from build123d import *

# Parameters (mm, degrees)
EXTRUDE_1_DEPTH          = 42.5
SKETCH_3_R               = 15
EXTRUDE_2_DEPTH          = 22
CUT_EXTRUDE_1_DEPTH      = 101.5
CUT_EXTRUDE_1_DEPTH_BACK = 101.5
FILLET_1_R               = 3
SKETCH_5_R               = 7.5
CUT_EXTRUDE_2_DEPTH      = 202


with BuildPart() as part:
    # 草图1 → 凸台-拉伸1 (new body, symmetric)
    with BuildSketch(Plane(origin=(0, 0, 0), x_dir=(0, 0, -1), z_dir=(1, 0, 0))):
        Polygon((-100.5, 100), (-42.5, 0), (42.5, 0), (100.5, 100), (100.5, 120), (95.5, 120), (95.5, 115), (95.5, 101.345066218), (39.619861593, 5), (-39.619861593, 5), (-95.5, 101.345066218), (-95.5, 115), (-95.5, 120), (-100.5, 120), align=None)
    extrude(amount=EXTRUDE_1_DEPTH, both=True)

    # 草图3 → 凸台-拉伸2 (add)
    with BuildSketch(Plane.XZ):
        Circle(SKETCH_3_R)
    extrude(amount=EXTRUDE_2_DEPTH)

    # 草图4 → 切除-拉伸1 (cut, two sides)
    with BuildSketch(Plane.XY) as cut_extrude_1_sk:
        Polygon((0, 78.450873214), (-15, 18.450873214), (15, 18.450873214), align=None)
    extrude(amount=CUT_EXTRUDE_1_DEPTH, mode=Mode.SUBTRACT)
    extrude(cut_extrude_1_sk.sketch, amount=-CUT_EXTRUDE_1_DEPTH_BACK, mode=Mode.SUBTRACT)

    # 圆角1
    fillet_1_edges = [part.edges().sort_by_distance(p)[0] for p in [
        (0, 78.450873214, -85.111437261),
        (0, 78.450873214, 85.111437261),
        (15, 18.450873214, -50.311437261),
        (15, 18.450873214, 50.311437261),
        (-15, 18.450873214, -50.311437261),
        (-15, 18.450873214, 50.311437261),
    ]]
    fillet(fillet_1_edges, radius=FILLET_1_R)

    # 草图5 → 切除-拉伸2 (cut, through all)
    with BuildSketch(Plane.XY.offset(100.5)):
        with Locations((0, 94)):
            Circle(SKETCH_5_R)
    extrude(amount=-CUT_EXTRUDE_2_DEPTH, mode=Mode.SUBTRACT)


solid = part.part
Input: part model. Units: mm. Frame: model coordinates. A direction names the side the tool comes from. Give positions to 0.01 mm unless a question says otherwise; leave off trailing zeros. Loops run counter-clockwise (first coordinate to the right, second up) from the corner with the lowest first, then second, coordinate; pieces in that order, holes last. Notation, with made-up numbers: (64, 69) -> (107, 69) arc R10 ccw to (107, 74) -> close; hole circle Ø7 at (17.5, 13.25). An arc over 180 degrees is marked (long way). Answer as a JSON object with one key per item and string values. Group by question number.
Item 1: Cut plane D-D, the plane x = 24. Return the cut outline in (y, z), and give its area (3 significant figures).
Item 2: Pin query (flat end, axial travel): P1, Ø1, axis at x = 24.5, z = 22, coming from the -Y side; P2, Ø1.5, axis at x = 25.5, y = 25, coming from the -Z side (3 decimals); P3, Ø3, axis at x = 13.5, y = 74, coming from the -Z side; P4, Ø12, axis at x = 0, y = 94, coming from the -Z side. Return the tip coordinate at first contact, or that it passes through.
Item 3: Reachability of faces 4 (the flat face through (1, 111, 95.5)), 5 (the cylindrical face through (6.93, 91.13, -93.55)) from +Z, -Z, +X, -X, +Y, -Y: full face, straight path, thin tool, end or side. Return the list, or none.
Item 4: Cut plane B-B, the plane z = 0. Return the cut outline in (x, y), and give its area (4 significant figures).
Item 5: Cut plane A-A, the plane y = 104.5. Return the cut outline in (x, z), and give its area (3 significant figures).
Item 6: Pull-direction query (Z, two-part tool) for faces 1 (the flat face through (1, 0, 19)), 2 (the flat face through (1, 110, 100.5)), 3 (the flat face through (10.039, 53.847, -67.951)); classes: released by +Z, released by -Z, zero draft, split by the parting line, or undercut.
Item 7: Cut plane C-C, the plane y = 52.5. Return the cut outline in (x, z).
Item 8: Line query: probe 1 along Z at (x, y) = (28.5, 111.5); probe 2 along X at (y, z) = (94, 96.25); probe 3 along Y at (x, z) = (7.5, 31). Output: solid intervals per line, ascending.
Checks:
{
 "1": {"outline": "(0, -42.5) -> (100, -100.5) -> (120, -100.5) -> (120, -95.5) -> (101.35, -95.5) -> (5, -39.62) -> (5, 39.62) -> (101.35, 95.5) -> (120, 95.5) -> (120, 100.5) -> (100, 100.5) -> (0, 42.5) -> close", "area": "1,740 mm²"},
 "2": {"P1": "stops at y = 0", "P2": "stops at z = -57.435", "P3": "stops at z = -86.29", "P4": "passes through"},
 "3": {"face 4": "+X, -X, +Y", "face 5": "+Z, -Z"},
 "4": {"outline": "(-42.5, 0) -> (-15, 0) -> (-15, -22) -> (15, -22) -> (15, 0) -> (42.5, 0) -> (42.5, 5) -> (-42.5, 5) -> close", "area": "1,085 mm²"},
 "5": {"outline": "(-42.5, -100.5) -> (42.5, -100.5) -> (42.5, -95.5) -> (-42.5, -95.5) -> close; (-42.5, 95.5) -> (42.5, 95.5) -> (42.5, 100.5) -> (-42.5, 100.5) -> close", "area": "850 mm²"},
 "6": {"face 1": "zero draft", "face 2": "released by +Z", "face 3": "undercut"},
 "7": {"outline": "(-42.5, -72.95) -> (-6.49, -72.95) -> (-6.49, -67.17) -> (-42.5, -67.17) -> close; (-42.5, 67.17) -> (-6.49, 67.17) -> (-6.49, 72.95) -> (-42.5, 72.95) -> close; (6.49, -72.95) -> (42.5, -72.95) -> (42.5, -67.17) -> (6.49, -67.17) -> close; (6.49, 67.17) -> (42.5, 67.17) -> (42.5, 72.95) -> (6.49, 72.95) -> close"},
 "8": {"probe 1": "z = -100.5 to -95.5, 95.5 to 100.5", "probe 2": "x = -42.5 to -7.5, 7.5 to 42.5", "probe 3": "y = 0 to 5"}
}
